Autodesk Fusion 360 part; units mm, degrees
sketch "Schizzo1" plane through (0, 0, 0) normal (0, 0, 1) x (1, 0, 0)
  line L0 (0, 0) -> (-25, 0)
  line L1 (-25, 0) -> (-25, 3)
  line L2 (-25, 3) -> (-5, 3)
  line L3 (-5, 3) -> (-5, 11.5)
  line L4 (-5, 11.5) -> (-25, 11.5)
  line L5 (-25, 11.5) -> (-25, 14.5)
  line L6 (-25, 14.5) -> (0, 14.5)
  line L7 (0, 14.5) -> (0, 0)
  line L8 (12.5574, 7.25) -> (25.0574, -14.4006)
  line L9 (12.4593, 1.4199) -> (5.0981, -2.8301)
  line L10 (0, 0) -> (12.5574, 7.25)
  line L11 (12.5, -21.6506) -> (0, 0)
  line L12 (5.0981, -2.8301) -> (15.0981, -20.1506)
  line L13 (25.0574, -14.4006) -> (22.4593, -15.9006)
  line L14 (15.0981, -20.1506) -> (12.5, -21.6506)
  line L15 (22.4593, -15.9006) -> (12.4593, 1.4199)
  line L16 (0, 14.5) -> (12.5574, 7.25)
  point P0 (12.5574, 7.25)
  dimension "d2" = 8.5
  dimension "d3" = 3
  dimension "d4" = 3
  dimension "d5" = 25
  dimension "d6" = 25
  dimension "d7" = 20
  dimension "d8" = 8.5
  dimension "d9" = 3
  dimension "d10" = 3
  dimension "d11" = 25
  dimension "d12" = 25
  dimension "d13" = 20
  dimension "d16" = 60
extrude "Estrusione1" add sketch "Schizzo1" along normal blind 250
fillet "Raccordo1" radius 5 1 edges at (0, 0, 125)
Here's how the part is built. I have some questions about the finished solid (model axes, mm). A direction names the side the tool comes from. Give positions to 0.01 mm unless a question says otherwise; leave off trailing zeros. Loops run counter-clockwise (first coordinate to the right, second up) from the corner with the lowest first, then second, coordinate; pieces in that order, holes last. Notation, with made-up numbers: (30, -8.75) -> (89, -8.75) arc R26 cw to (89, 11.25) -> close; hole circle Ø7 at (85, 76.25). An arc over 180 degrees is marked (long way). Use one line per item in the form item = value. Start each with the question number.
1) Please list where these lines run through material, in increasing order: line 1 along Y through (x, z) = (-20, 89); line 2 along Y through (x, z) = (6, 90.5); line 3 along X through (y, z) = (-3.5, 59).
2) Imagine slicing it at C-C (y = -11.5). Please give me the cut outline in (x, z), then the cut area to 3 significant figures.
3) Thinking about a two-plate mould opening in Y: for faces 5 (the face through (-13, 14.5, 123)), 6 (the face through (-15, 11.5, 123)), 7 (the face through (-0.355, -0.688, 126.75)), 8 (the face through (-5, 7, 123)), which applies, +Y half, -Y half, draft (parallel to the pull), parting line (faces both ways), or undercut?
4) Which directions (+Z, -Z, +X, -X, +Y, -Y) give clear straight access to the entire face, cutting with the end or side of a thin tool? Please do faces 1 (the face through (-15, 3, 123)), 2 (the face through (2, 2, 0)), 3 (the face through (10.03, -11.37, 123.25)), 4 (the face through (-14, 0, 123)).
5) Imagine slicing it at A-A (x = -16). Please give me the cut outline in (y, z).
6) For P1, Ø1.5, axis at y = 4.5, z = 128.5, coming from the +X side; P2, Ø4, axis at x = -13, z = 49.5, coming from the -Y side; P3, Ø10, axis at x = -13, y = 2, coming from the -Z side; P4, Ø5, axis at x = -8.5, y = 8, coming from the -Z side, each with a flat end and sliding along its axis, tell me the tip position at first contact or that it passes through.
7) Imagine slicing it at B-B (z = 42.5). Please give me the cut outline in (x, y), then the cut area to 3 significant figures.
Check values:
q1.line_1 = 0 to 3, 11.5 to 14.5
q1.line_2 = -10.39 to -4.39, -2.31 to 11.04
q1.line_3 = 2.02 to 5.48, 15.3 to 18.76
q2.outline = (6.64, 0) -> (10.1, 0) -> (10.1, 250) -> (6.64, 250) -> close; (19.92, 0) -> (23.38, 0) -> (23.38, 250) -> (19.92, 250) -> close
q2.area = 1,730 mm^2
q3.face_5 = +Y half
q3.face_6 = undercut
q3.face_7 = -Y half
q3.face_8 = undercut
q4.face_1 = +Z, -Z, -X
q4.face_2 = -Z, +X, -X, +Y, -Y
q4.face_3 = +Z, -Z
q4.face_4 = +Z, -Z, -X, -Y
q5.outline = (0, 0) -> (3, 0) -> (3, 250) -> (0, 250) -> close; (11.5, 0) -> (14.5, 0) -> (14.5, 250) -> (11.5, 250) -> close
q6.P1 = 14.58
q6.P2 = 0
q6.P3 = 0
q6.P4 = through
q7.outline = (-25, 0) -> (-2.89, 0) arc R5 cw to (1.44, -2.5) -> (12.5, -21.65) -> (15.1, -20.15) -> (5.1, -2.83) -> (12.46, 1.42) -> (22.46, -15.9) -> (25.06, -14.4) -> (12.56, 7.25) -> (0, 14.5) -> (-25, 14.5) -> (-25, 11.5) -> (-5, 11.5) -> (-5, 3) -> (-25, 3) -> close
q7.area = 477 mm^2
